The listing builds one solid part. Answer for the finished solid, in the listing's coordinates (mm). Coordinates: 2 decimals unless noted, no trailing zeros. Order: outer loops, then holes, each group sorted by start corner. A loop starts at its lowest first (then second) coordinate and runs counter-clockwise, first axis right, second up.
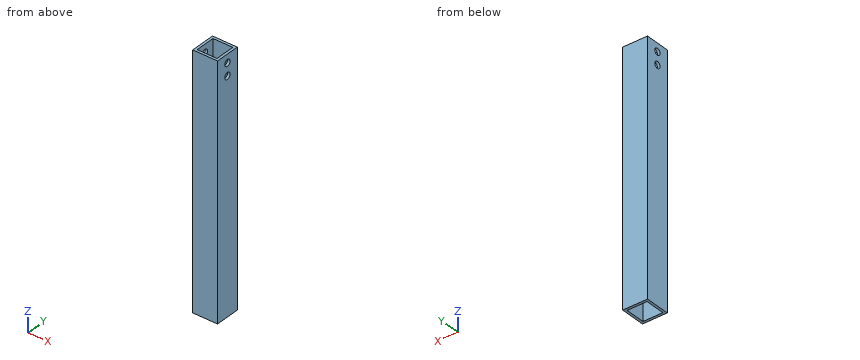
from build123d import *

# Parameters (mm, degrees)
F0_W     = 30
F0_H     = 30
F0_W_2   = 24
F0_H_2   = 24
F1_DEPTH = 150
F3_D     = 8


with BuildPart() as f1:
    # F0 (on Top) → F1 (new body, symmetric)
    with BuildSketch(Plane.XY):
        Rectangle(F0_W, F0_H)
        Rectangle(F0_W_2, F0_H_2, mode=Mode.SUBTRACT)
    extrude(amount=F1_DEPTH, both=True)

    # F3 (through all)
    with Locations(Plane.YZ.offset(15)):
        with Locations((0, 140), (0, 125)):
            Hole(F3_D / 2)


solid = f1.part
(1) Find section D-D on z = -56. Determine the outline of the cut face in (x, y), then the cut area to 3 significant figures.
(2) Given pin 1 Ø6.5 at (y, z) = (0, 125) entering from -X, flat-ended and moving along its own axis, determine where the tip first touches the part or whether it passes through.
(3) Find section B-B on x = -3.25. Determine the outline of the cut face in (y, z).
(4) Find the intervals of material crossed by probe 1 along Z at (x, y) = (-14, 0); probe 2 along Y at (x, z) = (5, -57), in increasing order.
(5) Find section A-A on z = 125. Determine the outline of the cut face in (x, y), then the cut area to 3 significant figures.
(6) Find section C-C on y = 0. Determine the outline of the cut face in (x, z), then the cut area to 3 significant figures.
Resolved:
1. outline: (-15, -15) - (15, -15) - (15, 15) - (-15, 15) - close; hole (-12, -12) - (12, -12) - (12, 12) - (-12, 12) - close
1. area: 324 mm2
2. pin 1: passes through
3. outline: (-15, -150) - (-12, -150) - (-12, 150) - (-15, 150) - close; (12, -150) - (15, -150) - (15, 150) - (12, 150) - close
4. probe 1: z = -150 to 121, 129 to 136, 144 to 150
4. probe 2: y = -15 to -12, 12 to 15
5. outline: (-15, -15) - (15, -15) - (15, -4) - (12, -4) - (12, -12) - (-12, -12) - (-12, -4) - (-15, -4) - close; (-15, 4) - (-12, 4) - (-12, 12) - (12, 12) - (12, 4) - (15, 4) - (15, 15) - (-15, 15) - close
5. area: 276 mm2
6. outline: (-15, -150) - (-12, -150) - (-12, 121) - (-15, 121) - close; (-15, 129) - (-12, 129) - (-12, 136) - (-15, 136) - close; (-15, 144) - (-12, 144) - (-12, 150) - (-15, 150) - close; (12, -150) - (15, -150) - (15, 121) - (12, 121) - close; (12, 129) - (15, 129) - (15, 136) - (12, 136) - close; (12, 144) - (15, 144) - (15, 150) - (12, 150) - close
6. area: 1,700 mm2
